```python
from build123d import *

# Parameters (mm, degrees)
SKETCH2_R          = 2
CUT_EXTRUDE3_DEPTH = 33.832910319


with BuildPart() as part:
    # Sketch1 → Revolve1 (revolve)
    with BuildSketch(Plane(origin=(0, 0, 0), x_dir=(0, 0, -1), z_dir=(1, 0, 0)), mode=Mode.PRIVATE) as revolve1_sk:
        Polygon((-7, 2), (-7, 5), (-3, 5), (-3, 19), (-7, 19), (-7, 21), (11, 21), (11, 15), (7, 15), (7, 2), align=None)
    revolve(revolve1_sk.sketch.rotate(Axis((0, 0, 6.263706564), (0, 0, -1)), 90), axis=Axis((0, 0, 6.263706564), (0, 0, -1)))

    # Sketch2 → Cut-Extrude3 (cut, through all)
    with BuildSketch(Plane(origin=(0, 0, -7), x_dir=(-1, 0, 0), z_dir=(0, 0, -1))):
        with Locations((0, 12)):
            Circle(SKETCH2_R)
        with Locations((10.392304845, 6)):
            Circle(SKETCH2_R)
        with Locations((10.392304845, -6)):
            Circle(SKETCH2_R)
        with Locations((0, -12)):
            Circle(SKETCH2_R)
        with Locations((-10.392304845, -6)):
            Circle(SKETCH2_R)
        with Locations((-10.392304845, 6)):
            Circle(SKETCH2_R)
    extrude(amount=-CUT_EXTRUDE3_DEPTH, mode=Mode.SUBTRACT)


solid = part.part
```
Source: CAD feature listing. Evaluate the final solid. Frame: model axes, mm. A direction names the side the tool comes from. Round coordinates to 2 decimals unless told otherwise and drop trailing zeros. Loops run counter-clockwise (first coordinate to the right, second up) from the corner with the lowest first, then second, coordinate; pieces in that order, holes last. Notation, with made-up numbers: M 50.5,64 L 97.5,64 A7 ccw 97.5,68 Z; hole C -35,57 d2. An arc over 180 degrees is marked long. Put each result on its own line as item: value.
(1) Section D-D, the plane x = 11.5. Return loops of the section in (y, z).
Solutions:
outline: M -17.57,-11 L -9.63,-11 L -9.63,-7 L -7.67,-7 L -7.67,3 L -15.12,3 L -15.12,7 L -17.57,7 Z; M -4.33,-7 L 4.33,-7 L 4.33,3 L -4.33,3 Z; M 7.67,-7 L 9.63,-7 L 9.63,-11 L 17.57,-11 L 17.57,7 L 15.12,7 L 15.12,3 L 7.67,3 Z
(2) Ray query, line 1 (Y direction, x = 0, z = -4.75); line 2 (Z direction, x = 7.5, y = 16); line 3 (Z direction, x = -6.5, y = -9.5). Return the intervals inside material, ascending. Write a range as [from, to].
Solutions:
line 1: [-21, -14], [-10, -2], [2, 10], [14, 21]
line 2: [-11, 3]
line 3: [-7, 3]
(3) Section C-C, the plane y = -6. Return loops of the section in (x, z).
Solutions:
outline: M -20.12,-11 L -13.75,-11 L -13.75,-7 L -12.39,-7 L -12.39,3 L -18.03,3 L -18.03,7 L -20.12,7 Z; M -8.39,-7 L 8.39,-7 L 8.39,3 L -8.39,3 Z; M 12.39,-7 L 13.75,-7 L 13.75,-11 L 20.12,-11 L 20.12,7 L 18.03,7 L 18.03,3 L 12.39,3 Z
(4) First-contact query: pin 1 (3 mm diameter, centred on x = -16.5, z = 3, fed in from +Y); pin 2 (9 mm diameter, centred on x = 4.5, y = -3, fed in from -Z); pin 3 (5 mm diameter, centred on x = 0, y = 12, fed in from +Z). Flat tips, straight axial feed; report the tip coordinate or a pass-through.
Solutions:
pin 1: y = 14.7
pin 2: z = -7
pin 3: z = 3
(5) Section A-A, the plane z = -0.25. Return loops of the section in (x, y), and give its area (3 significant figures).
Solutions:
outline: C 0,0 d42; hole C -10.39,-6 d4; hole C -10.39,6 d4; hole C 0,-12 d4; hole C 0,0 d4; hole C 0,12 d4; hole C 10.39,-6 d4; hole C 10.39,6 d4
area: 1,300 mm²
(6) Section B-B, the plane x = 0. Return loops of the section in (y, z).
Solutions:
outline: M -21,-11 L -15,-11 L -15,-7 L -14,-7 L -14,3 L -19,3 L -19,7 L -21,7 Z; M -10,-7 L -2,-7 L -2,7 L -5,7 L -5,3 L -10,3 Z; M 2,-7 L 10,-7 L 10,3 L 5,3 L 5,7 L 2,7 Z; M 14,-7 L 15,-7 L 15,-11 L 21,-11 L 21,7 L 19,7 L 19,3 L 14,3 Z
(7) Access query for faces 1 (the face through (-4.119, 18.548, 5.028)), 2 (the face through (0, 3, -7)), 3 (the face through (11.979, -7.217, -2.07)). Directions: +Z, -Z, +X, -X, +Y, -Y. A direction counts if a zero-diameter tool reaches every point of the face in a straight line with its end or side. Return the directions, or none.
Solutions:
face 1: +Z
face 2: -Z
face 3: +Z, -Z
(8) Pull-direction query (Y, two-part tool) for faces 4 (the face through (-8.394, 6.088, -2.07)), 5 (the face through (16, 11, 7)), 6 (the face through (20.03, -6.31, -2.13)); classes: released by +Y, released by -Y, zero draft, split by the parting line, or undercut.
Solutions:
face 4: undercut
face 5: zero draft
face 6: split by the parting line
